Check sheet for the modelled part. Datum: model origin and axes. Units: mm. Round coordinates to 2 decimals unless told otherwise and drop trailing zeros. Loops run counter-clockwise (first coordinate to the right, second up) from the corner with the lowest first, then second, coordinate; pieces in that order, holes last. Notation, with made-up numbers: M 84,46 L 90,46 A32 cw 90,75 Z; hole C 83.25,37 d10. An arc over 180 degrees is marked long. Write item = value, one per line. Start each with the question number.
(1) Cross-section at C-C on x = 50. Record the boundary of the cut face in (y, z).
(2) Scan lines: L1, parallel to Y at x = 11, z = 2.5; L2, parallel to Y at x = -95, z = 5.5; L3, parallel to X at y = 45.5, z = 3.85. Record each from-to range of solid material in increasing order. Write a range as from..to.
(3) Go/stop test with a flat-tipped pin: P1, Ø1.8, axis at x = -48, z = 3, coming from the -Y side. Record where the tip stops, or that it passes through.
(4) Cross-section at B-B on y = 12. Record the boundary of the cut face in (x, z).
(5) Cross-section at A-A on z = 3.9. State how many separate pieces and enclosed holes the cut face has, plus the area to 3 significant figures.
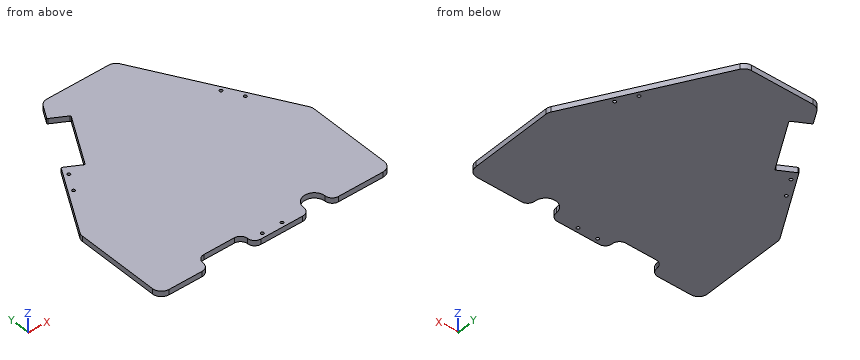
from build123d import *

# Parameters (mm, degrees)
F1_DEPTH = 6
F2_R     = 10
F3_R     = 7.99999
F5_D     = 3.3
F6_DEPTH = 6.001
F7_R     = 1


# Not quite as in the source:
# - a fillet or chamfer is up to 0.001 mm smaller than in the source, because OpenCascade refuses the exact size


with BuildPart() as f1:
    # F0 (on Top) → F1 (new body)
    with BuildSketch(Plane.XY):
        with BuildLine():
            Line((62, -130), (130, -130))
            Line((130, -130), (130, -25.455173281))
            Line((130, -25.455173281), (40.2479138593, 130))
            Line((40.2479138593, 130), (-40.2479138593, 130))
            Line((-40.2479138593, 130), (-130, -25.455173281))
            Line((-130, -25.455173281), (-130, -130))
            Line((-130, -130), (-75, -130))
            Line((-75, -130), (-75, -114))
            Line((-75, -114), (-25, -114))
            Line((-25, -114), (-25, -130))
            Line((-25, -130), (38, -130))
            Line((38, -130), (38, -122))
            ThreePointArc((38, -122), (50, -110), (62, -122))
            Line((62, -122), (62, -130))
        make_face()
    extrude(amount=F1_DEPTH)

    # F2
    f2_edges = [f1.edges().sort_by_distance(p)[0] for p in [
        (130, -25.455173, 3),
        (40.247914, 130, 3),
        (-40.247914, 130, 3),
        (-130, -25.455173, 3),
        (130, -130, 3),
        (-130, -130, 3),
    ]]
    fillet(f2_edges, radius=F2_R)

    # F3 (radius 8 in the source; OpenCascade refuses exactly that, so slightly less here)
    f3_edges = [f1.edges().sort_by_distance(p)[0] for p in [
        (-75, -130, 3),
        (-75, -114, 3),
        (-25, -114, 3),
        (-25, -130, 3),
        (38, -130, 3),
        (62, -130, 3),
    ]]
    fillet(f3_edges, radius=F3_R)

    # F5 (through all)
    with Locations(Plane.XY.offset(6)):
        with Locations((11, -125), (-11, -125), (-96.3493649054, 22.8294364099), (-85.3493649054, 41.8819952931), (96.3493649054, 22.8294364099), (85.3493649054, 41.8819952931)):
            Hole(F5_D / 2)

    # F4 (on face) → F6 (cut, through all)
    with BuildSketch(Plane.XY.offset(6)):
        Polygon((-51.6794919243, 110.1999259807), (-84.6794919243, 53.042249331), (-66.4929584448, 42.542249331), (-33.4929584448, 99.6999259807), align=None)
    extrude(amount=-F6_DEPTH, mode=Mode.SUBTRACT)

    # F7
    f7_edges = [f1.edges().sort_by_distance(p)[0] for p in [
        (-33.492958, 99.699926, 3),
        (-66.492958, 42.542249, 3),
        (-51.679492, 110.199926, 3),
        (-84.679492, 53.042249, 3),
    ]]
    fillet(f7_edges, radius=F7_R)


solid = f1.part
Result:
q1.outline = M -110,0 L 113.11,0 L 113.11,6 L -110,6 Z
q2.L1 = -130..-126.65, -123.35..130
q2.L2 = -130..21.88, 23.78..35.17
q2.L3 = -89.03..-71.62, -64.79..89.03
q3.P1 = -114
q4.outline = M -108.38,0 L 108.38,0 L 108.38,6 L -108.38,6 Z
q5.separate_pieces = 1
q5.enclosed_holes = 6
q5.area = 50,900 mm^2
